```python
from build123d import *

# Parameters (mm, degrees)
CORTE_EXTRUS_O1_DEPTH = 71


with BuildPart() as part:
    # Sketch1 → Revolve1 (revolve)
    with BuildSketch(Plane.XY):
        Polygon((70, -12.5), (0, -12.5), (0, -30), (10, -30), (12.679491924, -20), (22.320508076, -20), (25, -30), (35, -30), (35, -122.5), (45, -122.5), (47.679491924, -112.5), (57.320508076, -112.5), (60, -122.5), (70, -122.5), align=None)
    revolve(axis=Axis((0, 0, 0), (1, 0, 0)))

    # Esboço1 → Corte-extrusão1 (cut, through all)
    with BuildSketch(Plane.ZY):
        with BuildLine():
            Line((3.5, -16.5), (-3.5, -16.5))
            ThreePointArc((-3.5, -16.5), (-3.853553391, -16.353553391), (-4, -16))
            Line((-4, -16), (-4, -8.5))
            Line((-4, -8.5), (4, -8.5))
            Line((4, -8.5), (4, -16))
            ThreePointArc((4, -16), (3.853553391, -16.353553391), (3.5, -16.5))
        make_face()
    extrude(amount=-CORTE_EXTRUS_O1_DEPTH, mode=Mode.SUBTRACT)


solid = part.part
```
Here's how the part is built. I have some questions about the finished solid (model axes, mm). A direction names the side the tool comes from. Coordinates: 2 decimals unless noted, no trailing zeros. Loops run counter-clockwise (first coordinate to the right, second up) from the corner with the lowest first, then second, coordinate; pieces in that order, holes last. Notation, with made-up numbers: (89.25, -5) - (128.25, -5) arc R18 ccw to (128.25, 27) - close; hole circle Ø7 at (62.25, 12.5). An arc over 180 degrees is marked (long way). Return JSON: item names as keys, results as strings. Group by question number.
Item 1: Will these pins go through, and if not, where does the flat tip stop? P1, Ø1, axis at x = 37.5, z = -79.5, coming from the +Y side; P2, Ø3, axis at x = 41.5, z = 21, coming from the +Y side; P3, Ø1.5, axis at y = 26, z = -69.5, coming from the -X side.
Item 2: If we section it at B-B on x = 39: Write out the boundary of the cut face in (y, z), and give its area (3 significant figures).
Item 3: We'd pull the mould along X, two halves only. Please class faces 1 (the face through (57.49, 24.52, 110.44)), 2 (the face through (40.07, 26.556, 119.587)), 3 (the face through (12.55, 4.44, 20)), 4 (the face through (0, 13, 0)): +X half, -X half, draft (parallel to the pull), parting line (faces both ways), or undercut.
Item 4: If we section it at A-A on y = 0: Write out the boundary of the cut face in (x, z).
Item 5: I need wall thicknesses on line 1 (Z direction, x = 41, y = 0); line 2 (Z direction, x = 15, y = 0); line 3 (Y direction, x = 34, z = 0). Which ranges of each line are inside material? Lowest first, please. Write a range as from..to.
Item 6: If we section it at C-C on z = 0: Write out the boundary of the cut face in (x, y).
Item 7: If we section it at D-D on x = 18.5: Write out the boundary of the cut face in (y, z).
Item 8: On a 3-axis mill with a long thin cutter (end or side, diameter ignored), from which of +Z, -Z, +X, -X, +Y, -Y can I reach the whole of each face in a straight line? I mean faces 5 (the face through (70, -26, -2)), 6 (the face through (22.5, -19.1, 7.9)), 7 (the face through (30.07, 29.97, -1.32)), 8 (the face through (35, -16.5, 0)). Say none if no direction works.
Calculated:
{
 "1": {"P1": "stops at y = 93.62", "P2": "stops at y = 120.94", "P3": "stops at x = 35"},
 "2": {"outline": "circle Ø245 at (0, 0); hole (-16.5, -3.5) arc R0.5 ccw to (-16, -4) - (-11.84, -4) arc R12.5 ccw (long way) to (-11.84, 4) - (-16, 4) arc R0.5 ccw to (-16.5, 3.5) - close", "area": "46,600 mm^2"},
 "3": {"face 1": "undercut", "face 2": "draft", "face 3": "undercut", "face 4": "-X half"},
 "4": {"outline": "(0, -30) - (10, -30) - (12.68, -20) - (22.32, -20) - (25, -30) - (35, -30) - (35, -122.5) - (45, -122.5) - (47.68, -112.5) - (57.32, -112.5) - (60, -122.5) - (70, -122.5) - (70, -12.5) - (0, -12.5) - close; (0, 12.5) - (70, 12.5) - (70, 122.5) - (60, 122.5) - (57.32, 112.5) - (47.68, 112.5) - (45, 122.5) - (35, 122.5) - (35, 30) - (25, 30) - (22.32, 20) - (12.68, 20) - (10, 30) - (0, 30) - close"},
 "5": {"line 1": "z = -122.5..-12.5, 12.5..122.5", "line 2": "z = -20..-12.5, 12.5..20", "line 3": "y = -30..-16.5, 12.5..30"},
 "6": {"outline": "(0, -30) - (10, -30) - (12.68, -20) - (22.32, -20) - (25, -30) - (35, -30) - (35, -122.5) - (45, -122.5) - (47.68, -112.5) - (57.32, -112.5) - (60, -122.5) - (70, -122.5) - (70, -16.5) - (0, -16.5) - close; (0, 12.5) - (70, 12.5) - (70, 122.5) - (60, 122.5) - (57.32, 112.5) - (47.68, 112.5) - (45, 122.5) - (35, 122.5) - (35, 30) - (25, 30) - (22.32, 20) - (12.68, 20) - (10, 30) - (0, 30) - close"},
 "7": {"outline": "circle Ø40 at (0, 0); hole (-16.5, -3.5) arc R0.5 ccw to (-16, -4) - (-11.84, -4) arc R12.5 ccw (long way) to (-11.84, 4) - (-16, 4) arc R0.5 ccw to (-16.5, 3.5) - close"},
 "8": {"face 5": "+Z, -Z, +X, +Y, -Y", "face 6": "none", "face 7": "-X", "face 8": "+X, -X"}
}
